from build123d import *

# Parameters (mm, degrees)
SM_BASE_FLANGE_1_DEPTH = 2


# Sheet-metal steps are written as plain solids
with BuildPart() as part:
    # Sketch 1 → Базовая кромка1 (new body)
    with BuildSketch(Plane.XY):
        with BuildLine():
            Line((-28.388920969, 12), (-28.388920969, -12))
            ThreePointArc((-28.388920969, -12), (-27.510241313, -14.121320344), (-25.388920969, -15))
            Line((-25.388920969, -15), (1.611079031, -15))
            Line((1.611079031, -15), (1.611079031, -41.004699494))
            Line((1.611079031, -41.004699494), (14.502501119, -122.397935229))
            Line((14.502501119, -122.397935229), (-11.116749626, -130.722134398))
            ThreePointArc((-11.116749626, -130.722134398), (-12.862718215, -132.213332448), (-13.042868191, -134.50235493))
            Line((-13.042868191, -134.50235493), (-5.626460326, -157.327711321))
            ThreePointArc((-5.626460326, -157.327711321), (-4.135262277, -159.073679911), (-1.846239794, -159.253829887))
            Line((-1.846239794, -159.253829887), (23.832286146, -150.910371039))
            Line((23.832286146, -150.910371039), (37.544374419, -193.111839379))
            ThreePointArc((37.544374419, -193.111839379), (36.639549016, -196.320108259), (33.329233371, -196.711909935))
            Line((33.329233371, -196.711909935), (8.597245129, -184.110332509))
            ThreePointArc((8.597245129, -184.110332509), (-77.67448455, 14.217890909), (38.659903534, 196.545084972))
            Line((38.659903534, 196.545084972), (14.44017549, 122.004426694))
            Line((14.44017549, 122.004426694), (1.611079031, 41.004699494))
            Line((1.611079031, 41.004699494), (1.611079031, 15))
            Line((1.611079031, 15), (-25.388920969, 15))
            ThreePointArc((-25.388920969, 15), (-27.510241313, 14.121320344), (-28.388920969, 12))
        make_face()
    extrude(amount=-SM_BASE_FLANGE_1_DEPTH)


solid = part.part
Could you check a few things on this model? Use its own coordinates, in mm. A direction names the side the tool comes from. Coordinates: 2 decimals unless noted, no trailing zeros. Order: outer loops, then holes, each group sorted by start corner. A loop starts at its lowest first (then second) coordinate and runs counter-clockwise, first axis right, second up. Notation, with made-up numbers: (35.5, -19.5) -> (91.5, -19.5) arc R9 cw to (91.5, -15.5) -> close; hole circle Ø10 at (39.5, -29.5). An arc over 180 degrees is marked (long way). One line per item, written item: value. Start each with the question number.
1) I'm going to push flat-ended pins straight in: pin 1 (1 mm diameter, centred on x = -16.5, z = -1, fed in from +Y); pin 2 (1 mm diameter, centred on y = -34, z = -0.5, fed in from +X); pin 3 (0.6 mm diameter, centred on y = 4, z = -0.5, fed in from +X). Where does each tip first touch, or does it pass through?
2) We'd pull the mould along X, two halves only. Please class faces 4 (the flat face through (26.72, 159.8, -0.99)), 5 (the flat face through (-32, 3, 0)), 6 (the flat face through (-9.387, -145.755, -0.986)): +X half, -X half, draft (parallel to the pull), parting line (faces both ways), or undercut.
3) If I drill on L1, parallel to Y at x = -14, z = -0.95; L2, parallel to X at y = -176, z = -0.75; L3, parallel to X at y = 163.5, z = -1.25, over which ranges is the centre line in solid material (lowest first)? Write a range as [from, to].
4) Which directions (+Z, -Z, +X, -X, +Y, -Y) give clear straight access to the entire face, cutting with the end or side of a thin tool? Please do faces 1 (the flat face through (10.81, -155.14, -0.99)), 2 (the flat face through (7.967, -81.132, -0.986)), 3 (the flat face through (21.14, -190.5, -0.99)).
5) Imagine slicing it at B-B on y = 117.5. List the corners of the cut face in (x, z) for me.
6) Imagine slicing it at C-C on x = -45. List the corners of the cut face in (y, z) for me.
7) Imagine slicing it at A-A on z = -0.7. List the corners of the cut face in (x, y) for me.
Answer list:
1. pin 1: stops at y = 153.66
1. pin 2: stops at x = 1.61
1. pin 3: stops at x = -28.39
2. face 4: +X half
2. face 5: draft
2. face 6: undercut
3. L1: y = [-163.57, -15], [15, 155.76]
3. L2: x = [-1.06, 31.98]
3. L3: x = [-6.18, 27.92]
4. face 1: +Z, -Z
4. face 2: +Z, -Z, +X
4. face 3: +Z, -Z, -X, -Y
5. outline: (-43.77, -2) -> (13.73, -2) -> (13.73, 0) -> (-43.77, 0) -> close
6. outline: (-123.3, -2) -> (115.49, -2) -> (115.49, 0) -> (-123.3, 0) -> close
7. outline: (-28.39, -12) -> (-28.39, 12) arc R3 cw to (-25.39, 15) -> (1.61, 15) -> (1.61, 41) -> (14.44, 122) -> (38.66, 196.55) arc R230.16 ccw to (8.6, -184.11) -> (33.33, -196.71) arc R3 ccw to (37.54, -193.11) -> (23.83, -150.91) -> (-1.85, -159.25) arc R3 cw to (-5.63, -157.33) -> (-13.04, -134.5) arc R3 cw to (-11.12, -130.72) -> (14.5, -122.4) -> (1.61, -41) -> (1.61, -15) -> (-25.39, -15) arc R3 cw to start
